Input: part model. Units: mm. Frame: model coordinates. A direction names the side the tool comes from. Round coordinates to 2 decimals unless told otherwise and drop trailing zeros. Write each loop counter-clockwise with the first axis right and the second up, starting at its lowest first coordinate (ties: lowest second). Pieces come first, ordered by that corner, then holes. Notation, with made-up numbers: (47.25, 63.5) -> (89.25, 63.5) arc R18 cw to (89.25, 90.5) -> close; hole circle Ø7 at (-27, 29). An arc over 180 degrees is marked (long way). Use CSV: the item, a comma, the result in double quotes.
```python
from build123d import *

# Parameters (mm, degrees)
SKETCH_1_W               = 24
SKETCH_1_H               = 24
SKETCH_1_W_2             = 16
SKETCH_1_H_2             = 16
EXTRUDE_1_DEPTH          = 20
SKETCH_2_W               = 24
SKETCH_2_H               = 4.5
EXTRUDE_2_DEPTH          = 40
CUT_EXTRUDE_1_DEPTH      = 40
CUT_EXTRUDE_1_DEPTH_BACK = 40
SKETCH_3_R               = 2.8
SKETCH_6_W               = 4
SKETCH_6_H               = 40
EXTRUDE_3_DEPTH          = 15.5
CHAMFER_1_SIZE           = 40
CHAMFER_1_SIZE2          = 14.558809371
SKETCH_7_R               = 5
CUT_EXTRUDE_2_DEPTH      = 1


with BuildPart() as part:
    # 草图1 → 凸台-拉伸1 (new body)
    with BuildSketch(Plane(origin=(0, 0, 0), x_dir=(1, 0, 0), z_dir=(0, 1, 0))):
        with Locations((8, 8)):
            Rectangle(SKETCH_1_W, SKETCH_1_H)
        with Locations((8, 8)):
            Rectangle(SKETCH_1_W_2, SKETCH_1_H_2, mode=Mode.SUBTRACT)
    extrude(amount=EXTRUDE_1_DEPTH)

    # 草图2 → 凸台-拉伸2 (add)
    with BuildSketch(Plane.XY.offset(4)):
        with Locations((8, 17.75)):
            Rectangle(SKETCH_2_W, SKETCH_2_H)
    extrude(amount=EXTRUDE_2_DEPTH)

    # 草图3 → 切除-拉伸1 (cut, two sides: drawn at the far end of the back side and taken through both)
    with BuildSketch(Plane(origin=(0, 15.5, 0), x_dir=(-1, 0, 0), z_dir=(0, -1, 0)).offset(-CUT_EXTRUDE_1_DEPTH_BACK)):
        with Locations(Location((-8, -37, 0), (0, 0, 270))):
            Circle(SKETCH_3_R)
    extrude(amount=CUT_EXTRUDE_1_DEPTH + CUT_EXTRUDE_1_DEPTH_BACK, mode=Mode.SUBTRACT)

    # 草图6 → 凸台-拉伸3 (add)
    with BuildSketch(Plane(origin=(0, 15.5, 0), x_dir=(-1, 0, 0), z_dir=(0, -1, 0))):
        with Locations((-1, -24)):
            Rectangle(SKETCH_6_W, SKETCH_6_H)
        with Locations((-15, -24)):
            Rectangle(SKETCH_6_W, SKETCH_6_H)
    extrude(amount=EXTRUDE_3_DEPTH)

    # 倒角1
    chamfer_1_edges = [part.edges().sort_by_distance(p)[0] for p in [
        (1, 0, 44),
        (15, 0, 44),
    ]]
    chamfer_1_side = [part.faces().sort_by_distance(p)[0] for p in [
        (-3.3164797, 0, -8),
    ]]
    chamfer(chamfer_1_edges, length=CHAMFER_1_SIZE, length2=CHAMFER_1_SIZE2, reference=chamfer_1_side[0])

    # 草图7 → 切除-拉伸2 (cut)
    with BuildSketch(Plane(origin=(0, 15.5, 0), x_dir=(-1, 0, 0), z_dir=(0, -1, 0))):
        with Locations(Location((-8, -37, 0), (0, 0, 90))):
            Circle(SKETCH_7_R)
    extrude(amount=-CUT_EXTRUDE_2_DEPTH, mode=Mode.SUBTRACT)


solid = part.part
```
Item 1: Pull-direction query (Z, two-part tool) for faces 4 (the face through (8, 17, 44)), 5 (the face through (20, 12, -3)), 6 (the face through (5.8, 16.5, 34.8)); classes: +Z half, -Z half, draft (parallel to the pull), parting line (faces both ways), or undercut.
Worked answers:
face 4,"+Z half"
face 5,"draft"
face 6,"undercut"
Item 2: Section query D-D on x = 8. Return the cut outline in (y, z), plus the area to 3 significant figures.
Worked answers:
outline,"(0, -20) -> (20, -20) -> (20, -16) -> (0, -16) -> close; (0, 0) -> (20, 0) -> (20, 34.2) -> (16.5, 34.2) -> (16.5, 32) -> (15.5, 32) -> (15.5, 4) -> (0, 4) -> close; (15.5, 42) -> (16.5, 42) -> (16.5, 39.8) -> (20, 39.8) -> (20, 44) -> (15.5, 44) -> close"
area,"310 mm²"
Item 3: Line query: line 1 (Z direction, x = 8, y = 16); line 2 (Z direction, x = 8.25, y = 12.75); line 3 (X direction, y = 11.5, z = 32). Output: solid intervals per line, ascending.
Worked answers:
line 1,"z = -20 to -16, 0 to 32, 42 to 44"
line 2,"z = -20 to -16, 0 to 4"
line 3,"x = -1 to 3, 13 to 17"
Item 4: Section query C-C on x = 1.75. Return the cut outline in (y, z), plus the area to 3 significant figures.
Worked answers:
outline,"(0, -20) -> (20, -20) -> (20, -16) -> (0, -16) -> close; (0, 0) -> (20, 0) -> (20, 44) -> (14.56, 44) -> (0, 4) -> close"
area,"669 mm²"
Item 5: Set-up query: faces 1 (the face through (8, 15.5, 43)), 2 (the face through (8, 16, 42)), 3 (the face through (8, 10, 0)). Return all of +Z, -Z, +X, -X, +Y, -Y with unobstructed straight access to the full face (end or side cutting, diameter ignored); none if empty.
Worked answers:
face 1,"+Z, -Y"
face 2,"-Y"
face 3,"+Y, -Y"
Item 6: Section query A-A on y = 18.25. Return the cut outline in (x, z).
Worked answers:
outline,"(-4, -20) -> (20, -20) -> (20, 44) -> (-4, 44) -> close; hole (0, -16) -> (16, -16) -> (16, 0) -> (0, 0) -> close; hole circle Ø5.6 at (8, 37)"
Item 7: First-contact query: pin 1 Ø3.5 at (x, z) = (-2.5, 21) entering from -Y; pin 2 Ø3.5 at (x, z) = (8.5, 41.5) entering from -Y; pin 3 Ø1.5 at (x, y) = (18, 6.5) entering from +Z. Flat tips, straight axial feed; report the tip coordinate or a pass-through.
Worked answers:
pin 1,"stops at y = 5.86"
pin 2,"stops at y = 15.5"
pin 3,"stops at z = 4"
Item 8: Section query B-B on z = -11. Return the cut outline in (x, y), plus the area to 3 significant figures.
Worked answers:
outline,"(-4, 0) -> (0, 0) -> (0, 20) -> (-4, 20) -> close; (16, 0) -> (20, 0) -> (20, 20) -> (16, 20) -> close"
area,"160 mm²"
